Could you check a few things on this model? Use its own coordinates, in mm. A direction names the side the tool comes from. Coordinates: 2 decimals unless noted, no trailing zeros. Loops run counter-clockwise (first coordinate to the right, second up) from the corner with the lowest first, then second, coordinate; pieces in that order, holes last. Notation, with made-up numbers: (34.5, 50.25) -> (65.5, 50.25) arc R20 ccw to (65.5, 57.25) -> close; hole circle Ø6 at (-39.5, 14.25). An arc over 180 degrees is marked (long way). One line per question, with ' | ' between items.
from build123d import *

# Parameters (mm, degrees)
SKETCH1_W               = 190.5
SKETCH1_H               = 88.9
BOSS_EXTRUDE1_DEPTH     = 6.35
SKETCH2_W               = 5.588
SKETCH2_H               = 30.48
HOLE_DEPTH              = 6.35
SKETCH3_W               = 38.1
SKETCH3_H               = 6.35
TAB1_DEPTH              = 6.35
SKETCH4_W               = 38.1
SKETCH4_H               = 6.35
TAB2_DEPTH              = 6.35
SKETCH5_W               = 5.588
SKETCH5_H               = 5.588
DOWEL1_DEPTH            = 6.35
MIRROR2_COPY_1_SKETCH_W = 5.588
MIRROR2_COPY_1_SKETCH_H = 5.588
MIRROR2_COPY_1_DEPTH    = 6.35
SKETCH6_W               = 19.05
SKETCH6_H               = 5.588
SKETCH6_H_2             = 6.35
CUT_EXTRUDE1_DEPTH      = 7.35


with BuildPart() as part:
    # Sketch1 → Boss-Extrude1 (new body)
    with BuildSketch(Plane(origin=(0, 0, 0), x_dir=(1, 0, 0), z_dir=(0, 1, 0))):
        Rectangle(SKETCH1_W, SKETCH1_H)
    extrude(amount=BOSS_EXTRUDE1_DEPTH)

    # Sketch2 → hole (cut)
    with BuildSketch(Plane(origin=(0, 6.35, 0), x_dir=(1, 0, 0), z_dir=(0, 1, 0))):
        with Locations((-60.96, 0)):
            Rectangle(SKETCH2_W, SKETCH2_H)
        with Locations((-25.4, 0)):
            Rectangle(SKETCH2_W, SKETCH2_H)
        with Locations((10.16, 0)):
            Rectangle(SKETCH2_W, SKETCH2_H)
        with Locations((45.72, 0)):
            Rectangle(SKETCH2_W, SKETCH2_H)
    extrude(amount=-HOLE_DEPTH, mode=Mode.SUBTRACT)

    # Sketch3 → tab1 (add)
    with BuildSketch(Plane.ZY.offset(95.25)):
        with Locations((0, 3.175)):
            Rectangle(SKETCH3_W, SKETCH3_H)
    extrude(amount=TAB1_DEPTH)

    # Sketch4 → tab2 (add)
    with BuildSketch(Plane(origin=(95.25, 0, 0), x_dir=(0, 0, -1), z_dir=(1, 0, 0))):
        with Locations((0, 3.175)):
            Rectangle(SKETCH4_W, SKETCH4_H)
    extrude(amount=TAB2_DEPTH)

    # Sketch5 → dowel1 (cut)
    with BuildSketch(Plane(origin=(0, 6.35, 0), x_dir=(1, 0, 0), z_dir=(0, 1, 0))):
        with Locations((-79.756, 28.956)):
            Rectangle(SKETCH5_W, SKETCH5_H)
    dowel1 = extrude(amount=-DOWEL1_DEPTH, mode=Mode.SUBTRACT)

    # Mirror1: dowel1 across plane
    add(dowel1.mirror(Plane(origin=(0, 0, 0), x_dir=(0, 0, 1), z_dir=(1, 0, 0))), mode=Mode.SUBTRACT)

    # Mirror2: dowel1 across plane
    add(dowel1.mirror(Plane.XY), mode=Mode.SUBTRACT)

    # Mirror2 copy 1 sketch → Mirror2 copy 1 (cut)
    with BuildSketch(Plane(origin=(0, 6.35, 0), x_dir=(-1, 0, 0), z_dir=(0, 1, 0))):
        with Locations((-79.756, 28.956)):
            Rectangle(MIRROR2_COPY_1_SKETCH_W, MIRROR2_COPY_1_SKETCH_H)
    extrude(amount=-MIRROR2_COPY_1_DEPTH, mode=Mode.SUBTRACT)

    # Sketch6 → Cut-Extrude1 (cut, through all)
    with BuildSketch(Plane(origin=(0, 6.35, 0), x_dir=(1, 0, 0), z_dir=(0, 1, 0))):
        with Locations((-85.725, -41.656)):
            Rectangle(SKETCH6_W, SKETCH6_H)
        with Locations((85.725, -41.656)):
            Rectangle(SKETCH6_W, SKETCH6_H)
        with Locations((-85.725, 41.275)):
            Rectangle(SKETCH6_W, SKETCH6_H_2)
        with Locations((85.725, 41.275)):
            Rectangle(SKETCH6_W, SKETCH6_H_2)
    extrude(amount=-CUT_EXTRUDE1_DEPTH, mode=Mode.SUBTRACT)


solid = part.part
1) If we section it at A-A on z = -9.5: Please give me the cut outline in (x, y), and give its area (3 significant figures).
Data:
outline: (-101.6, 0) -> (-63.75, 0) -> (-63.75, 6.35) -> (-101.6, 6.35) -> close; (-58.17, 0) -> (-28.19, 0) -> (-28.19, 6.35) -> (-58.17, 6.35) -> close; (-22.61, 0) -> (7.37, 0) -> (7.37, 6.35) -> (-22.61, 6.35) -> close; (12.95, 0) -> (42.93, 0) -> (42.93, 6.35) -> (12.95, 6.35) -> close; (48.51, 0) -> (101.6, 0) -> (101.6, 6.35) -> (48.51, 6.35) -> close | area: 1,150 mm²
2) I need wall thicknesses on line 1 along X through (y, z) = (2, -0.5); line 2 along Z through (x, y) = (-81, 4.5); line 3 along X through (y, z) = (2.5, -30). Which ranges of each line are inside material? Lowest first, please. Write a range as from..to.
Data:
line 1: -101.6..-63.75, -58.17..-28.19, -22.61..7.37, 12.95..42.93, 48.51..101.6 | line 2: -38.1..-31.75, -26.16..26.16, 31.75..38.86 | line 3: -95.25..-82.55, -76.96..76.96, 82.55..95.25
3) I'm going to push flat-ended pins straight in: pin 1 Ø1.7 at (x, y) = (-80, 3) entering from +Z; pin 2 Ø3 at (y, z) = (2.5, -29.5) entering from +X. Where does each tip first touch, or does it pass through?
Data:
pin 1: z = 38.86 | pin 2: x = 95.25
4) If we section it at C-C on x = -86.5: Please give me the cut outline in (y, z).
Data:
outline: (0, -38.1) -> (6.35, -38.1) -> (6.35, 38.86) -> (0, 38.86) -> close
5) If we section it at B-B on y = 4: Give the number of separate pieces and of enclosed holes in the cut face, and give its area (3 significant figures).
Data:
separate pieces: 1 | enclosed holes: 8 | area: 16,200 mm²
6) On a 3-axis mill with a long thin cutter (end or side, diameter ignored), from which of +Z, -Z, +X, -X, +Y, -Y can I reach the whole of each face in a straight line? I mean faces 1 (the face through (-98, 3, 19.05)), 2 (the face through (86, 3, -38.1)), 3 (the face through (-80, 3, -26.162)). Say none if no direction works.
Data:
face 1: +Z, -X, +Y, -Y | face 2: -Z, +X, +Y, -Y | face 3: +Y, -Y
7) We'd pull the mould along X, two halves only. Please class faces 4 (the face through (101.6, 3, 0)), 5 (the face through (-86, 3, -38.1)), 6 (the face through (-63.754, 3, 0)): pulls with the +X half, pulls with the -X half, needs draft (parallel to the pull), parting line crosses it, or undercut.
Data:
face 4: pulls with the +X half | face 5: needs draft | face 6: undercut
